Work out the finished part from the listing and answer in its coordinate system (mm). Round coordinates to 2 decimals unless told otherwise and drop trailing zeros. Loops run counter-clockwise (first coordinate to the right, second up) from the corner with the lowest first, then second, coordinate; pieces in that order, holes last.
```python
from build123d import *

# Parameters (mm, degrees)
SKETCH1_R           = 3.175
SKETCH1_R_2         = 4.7625
BOSS_EXTRUDE1_DEPTH = 6.35
FILLET1_R           = 5


with BuildPart() as part:
    # Sketch1 → Boss-Extrude1 (new body)
    with BuildSketch(Plane.XY):
        Polygon((16.184070214, -255.902577388), (-19.05, -235.560177465), (-19.05, -178.2), (19.05, -178.2), (19.05, -255.902577388), align=None)
        with Locations((13.834070214, -246.4)):
            Circle(SKETCH1_R, mode=Mode.SUBTRACT)
        with Locations((-11.43, -231.16)):
            Circle(SKETCH1_R, mode=Mode.SUBTRACT)
        with Locations((0, -203.2)):
            Circle(SKETCH1_R_2, mode=Mode.SUBTRACT)
        with Locations((-11.43, -184.7)):
            Circle(SKETCH1_R, mode=Mode.SUBTRACT)
        with Locations((11.43, -184.7)):
            Circle(SKETCH1_R, mode=Mode.SUBTRACT)
    extrude(amount=BOSS_EXTRUDE1_DEPTH)

    # Fillet1
    fillet1_edges = [part.edges().sort_by_distance(p)[0] for p in [
        (-19.05, -235.560177465, 3.175),
        (-19.05, -178.2, 3.175),
        (19.05, -178.2, 3.175),
    ]]
    fillet(fillet1_edges, radius=FILLET1_R)


solid = part.part
```
1. Find section D-D (z = 1.75). Give the number of separate pieces and of enclosed holes in the cut face, then the cut area to 3 significant figures.
Answer key:
separate pieces: 1
enclosed holes: 5
area: 2,390 mm2
2. Find section A-A (y = -203.2). Write down the section's boundary in (x, z), then the cut area to 3 significant figures.
Answer key:
outline: (-19.05, 0) - (-4.76, 0) - (-4.76, 6.35) - (-19.05, 6.35) - close; (4.76, 0) - (19.05, 0) - (19.05, 6.35) - (4.76, 6.35) - close
area: 181 mm2
3. Find section B-B (x = 0). Write down the section's boundary in (y, z).
Answer key:
outline: (-246.56, 0) - (-207.96, 0) - (-207.96, 6.35) - (-246.56, 6.35) - close; (-198.44, 0) - (-178.2, 0) - (-178.2, 6.35) - (-198.44, 6.35) - close
4. Find section C-C (y = -184.7). Write down the section's boundary in (x, z) (3 decimals), then the cut area to 3 significant figures.
Answer key:
outline: (-19.05, 0) - (-14.605, 0) - (-14.605, 6.35) - (-19.05, 6.35) - close; (-8.255, 0) - (8.255, 0) - (8.255, 6.35) - (-8.255, 6.35) - close; (14.605, 0) - (19.05, 0) - (19.05, 6.35) - (14.605, 6.35) - close
area: 161 mm2
5. Consider probe 1 along X at (y, z) = (-184.7, 2.5) (3 decimals); probe 2 along Y at (x, z) = (-11.43, 4) (3 decimals); probe 3 along Y at (x, z) = (-9, 5). Determine where each line is inside the solid, lowest interval first.
Answer key:
probe 1: x = -19.05 to -14.605, -8.255 to 8.255, 14.605 to 19.05
probe 2: y = -239.96 to -234.335, -227.985 to -187.875, -181.525 to -178.2
probe 3: y = -241.36 to -233.2, -229.12 to -186.74, -182.66 to -178.2
6. Determine the mould class of faces 1 (the face through (-17.62, -179.7, 3.22)), 2 (the face through (11.02, -181.55, 3.13)), 3 (the face through (0, -217, 6.35)) for opening direction Y: +Y half, -Y half, draft (parallel to the pull), parting line (faces both ways), or undercut.
Answer key:
face 1: +Y half
face 2: undercut
face 3: draft
7. Given pin 1 (1.5 mm diameter, centred on x = -9.5, z = 4.5, fed in from -Y), flat-ended and moving along its own axis, determine where the tip first touches the part or whether it passes through.
Answer key:
pin 1: stops at y = -241.51
